Autodesk Inventor part; units mm, degrees
ref_plane "YZ Plane" through (0, 0, 0) normal (1, 0, 0) x (0, 1, 0)
ref_plane "XZ Plane" through (0, 0, 0) normal (0, 1, 0) x (-1, 0, 0)
ref_plane "XY Plane" through (0, 0, 0) normal (0, 0, 1) x (1, 0, 0)
sketch "Sketch1" plane through (0, 0, 0) normal (0, 0, 1) x (1, 0, 0)
  line L0 (0, 0) -> (42, 0)
  line L1 (42, 0) -> (42, 42)
  line L2 (42, 42) -> (0, 42)
  line L3 (0, 42) -> (0, 0)
  dimension "d0" = 42
  dimension "d1" = 42
extrude "Extrusion1" add sketch "Sketch1" along normal blind 9.5
chamfer "Chamfer1" distance 4.5 angle 45 4 edges at (0, 0, 4.75) (42, 0, 4.75) (42, 42, 4.75) (0, 42, 4.75)
sketch "Sketch6" plane through (0, 0, 0) normal (0, 0, -1) x (-1, 0, 0)
  line L0 (-42, 4.5) -> (-42, 37.5)
  line L1 (-4.5, 0) -> (-37.5, 0)
  circle A0 centre (-21, 21) radius 25.25
  dimension "d37" = 50.5
  dimension "d38" = 21
  dimension "d39" = 21
extrude "Extrusion5" cut sketch "Sketch6" against normal blind 2
sketch "Sketch2" plane through (0, 0, 9.5) normal (0, 0, 1) x (1, 0, 0)
  line L0 (4.5, 42) -> (37.5, 42)
  line L1 (0, 4.5) -> (0, 37.5)
  line L2 (37.5, 0) -> (4.5, 0)
  line L3 (42, 37.5) -> (42, 4.5)
  line L4 (10, 0) -> (10, 6)
  line L5 (10, 36) -> (10, 42)
  line L6 (0, 32) -> (6, 32)
  line L7 (36, 32) -> (42, 32)
  line L8 (0, 10) -> (6, 10)
  line L9 (36, 10) -> (42, 10)
  line L10 (32, 42) -> (32, 36)
  line L11 (32, 6) -> (32, 0)
  arc A0 (6, 32) -> (10, 36) centre (6, 36) ccw
  arc A1 (32, 36) -> (36, 32) centre (36, 36) ccw
  arc A2 (36, 10) -> (32, 6) centre (36, 6) ccw
  arc A3 (10, 6) -> (6, 10) centre (6, 6) ccw
  dimension "d10" = 4
extrude "Extrusion6" add sketch "Sketch2" along normal blind 2.5
fillet "Fillet3" radius 0.5 35 edges at (2.25, 2.25, 9.5) (7.25, 0, 9.5) (0, 7.25, 9.5) (34.75, 0, 9.5) (39.75, 2.25, 9.5) (42, 7.25, 9.5) (42, 34.75, 9.5) (34.75, 42, 9.5) (39.75, 39.75, 9.5) (0, 34.75, 9.5) (2.25, 39.75, 9.5) (7.25, 42, 9.5) (0, 21, 12) (42, 21, 12) (3, 10, 12) (8.8284, 8.8284, 12) (10, 3, 12) (21, 0, 12) (32, 3, 12) (33.1716, 8.8284, 12) (39, 10, 12) (33.1716, 33.1716, 12) (39, 32, 12) (32, 39, 12) (8.8284, 33.1716, 12) (10, 39, 12) (3, 32, 12) (21, 42, 12) (10, 0, 10.75) (32, 0, 10.75) (42, 10, 10.75) (42, 32, 10.75) (32, 42, 10.75) (10, 42, 10.75) (0, 32, 10.75)
sketch "Sketch7" plane through (0, 0, 12) normal (0, 0, 1) x (1, 0, 0)
  circle A0 centre (21, 21) radius 4.5
  line L0 (31.5, 42) -> (10.5, 42)
  line L1 (0, 31.5) -> (0, 10)
  dimension "d45" = 9
  dimension "d46" = 21
  dimension "d47" = 21
extrude "Extrusion7" cut sketch "Sketch7" against normal blind 3.5
fillet "Fillet4" radius 0.5 1 edges at (16.5, 21, 12)
sketch "Sketch8" plane through (0, 0, 9.5) normal (0, 0, 1) x (1, 0, 0)
  arc A0 (10, 6) -> (6, 10) centre (6, 6) ccw
  point P0 (36, 6)
  point P1 (6, 36)
  point P2 (36, 36)
  dimension "d51" = 30
  dimension "d52" = 30
hole "Hole2" at (6, 6, 9.5) at (36, 6, 9.5) at (6, 36, 9.5) at (36, 36, 9.5) direction (0, 0, -1) diameter 3 depth 5
properties part number "stepper_front"
Input: part model. Units: mm. Frame: model coordinates. A direction names the side the tool comes from. Coordinates: 2 decimals unless noted, no trailing zeros. Order: outer loops, then holes, each group sorted by start corner. A loop starts at its lowest first (then second) coordinate and runs counter-clockwise, first axis right, second up. Notation, with made-up numbers: (50, 82) - (80, 82) arc R16 cw to (80, 101) - close; hole circle Ø7 at (0.5, -32). An arc over 180 degrees is marked (long way). Put each result on its own line as item: value.
1. Cut plane A-A on z = 6.5. Return the cut outline in (x, y), then the cut area to 3 significant figures.
Report:
outline: (0, 4.5) - (4.5, 0) - (37.5, 0) - (42, 4.5) - (42, 37.5) - (37.5, 42) - (4.5, 42) - (0, 37.5) - close; hole circle Ø3 at (6, 6); hole circle Ø3 at (6, 36); hole circle Ø3 at (36, 6); hole circle Ø3 at (36, 36)
area: 1,700 mm2
2. Draft query along X for faces 1 (the face through (10, 39, 10)), 2 (the face through (21, 0, 6)), 3 (the face through (6, 6, 4.5)), 4 (the face through (3.19, 3.1, 0.99)). Return one class per face: pulls with the +X half, pulls with the -X half, needs draft (parallel to the pull), parting line crosses it, or undercut.
Report:
face 1: pulls with the -X half
face 2: needs draft
face 3: undercut
face 4: undercut
3. Cut plane C-C on x = 21. Return the cut outline in (y, z), then the cut area to 3 significant figures.
Report:
outline: (0, 2) - (42, 2) - (42, 11.5) arc R0.5 ccw to (41.5, 12) - (26, 12) arc R0.5 ccw to (25.5, 11.5) - (25.5, 8.5) - (16.5, 8.5) - (16.5, 11.5) arc R0.5 ccw to (16, 12) - (0.5, 12) arc R0.5 ccw to (0, 11.5) - close
area: 388 mm2
4. Contact query for flat-ended pins moving along their axis: pin 1 Ø1.6 at (y, z) = (38.5, 10.5) entering from +X; pin 2 Ø0.6 at (x, z) = (40, 10.5) entering from +Y; pin 3 Ø10.5 at (x, y) = (21, 21) entering from -Z. Output: stop coordinate, or through.
Report:
pin 1: stops at x = 32
pin 2: stops at y = 32
pin 3: stops at z = 2
5. Cut plane D-D on y = 14.5. Return the cut outline in (x, z), then the cut area to 3 significant figures.
Report:
outline: (0, 2) - (42, 2) - (42, 11.5) arc R0.5 ccw to (41.5, 12) - (0.5, 12) arc R0.5 ccw to (0, 11.5) - close
area: 420 mm2
6. Line query: line 1 along X through (y, z) = (6, 5.9); line 2 along X through (y, z) = (35, 6). Output: solid intervals per line, ascending.
Report:
line 1: x = 0 to 4.5, 7.5 to 34.5, 37.5 to 42
line 2: x = 0 to 4.88, 7.12 to 34.88, 37.12 to 42
7. Reachability of faces 5 (the face through (36.9, 37.2, 7)), 6 (the face through (3, 32, 10)), 7 (the face through (37, 4, 9.5)), 8 (the face through (4, 5, 9.5)), 9 (the face through (38.81, 38.9, 0.99)) from +Z, -Z, +X, -X, +Y, -Y: full face, straight path, thin tool, end or side. Return the list, or none.
Report:
face 5: +Z
face 6: +Z, -X, +Y
face 7: +Z, +X, -Y
face 8: +Z, -X, -Y
face 9: -Z
8. Cut plane B-B on z = 10.75. Return the cut outline in (x, y).
Report:
outline: (0, 10) - (6, 10) arc R4 cw to (10, 6) - (10, 0.5) arc R0.5 ccw to (10.5, 0) - (31.5, 0) arc R0.5 ccw to (32, 0.5) - (32, 6) arc R4 cw to (36, 10) - (41.5, 10) arc R0.5 ccw to (42, 10.5) - (42, 31.5) arc R0.5 ccw to (41.5, 32) - (36, 32) arc R4 cw to (32, 36) - (32, 41.5) arc R0.5 ccw to (31.5, 42) - (10.5, 42) arc R0.5 ccw to (10, 41.5) - (10, 36) arc R4 cw to (6, 32) - (0.5, 32) arc R0.5 ccw to (0, 31.5) - close; hole circle Ø9 at (21, 21)
